The figure shows three views and two pictorial views of one solid part (mm, origin at its lowest corner). Answer the questions. A direction names the side the tool comes from. Coordinates: 2 decimals unless noted, no trailing zeros. Write each loop counter-clockwise with the first axis right and the second up, starting at its lowest first coordinate (ties: lowest second). Pieces come first, ordered by that corner, then holes.
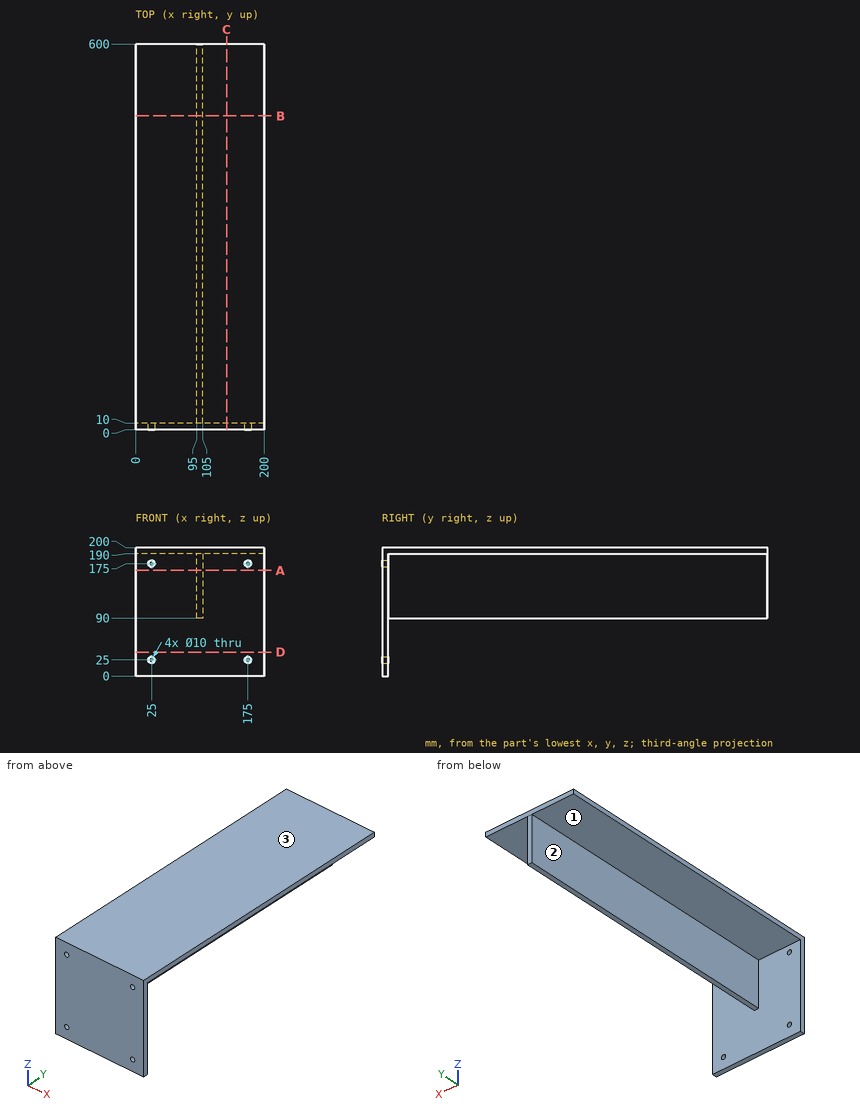
Q1. The part is cut by section B-B, the plane y = 488. Write down the section's boundary in (x, z).
Answers below:
outline: (0, 190) - (95, 190) - (95, 90) - (105, 90) - (105, 190) - (200, 190) - (200, 200) - (0, 200) - close
Q2. Find the intervals of material crossed by probe 1 along Z at (x, y) = (25, 9.8); probe 2 along Y at (x, z) = (163, 98), in increasing order.
Answers below:
probe 1: z = 0 to 20, 30 to 170, 180 to 200
probe 2: y = 0 to 10
Q3. The part is cut by section C-C, the plane x = 142. Write down the section's boundary in (y, z), then the cut area to 3 significant figures.
Answers below:
outline: (0, 0) - (10, 0) - (10, 190) - (600, 190) - (600, 200) - (0, 200) - close
area: 7,900 mm2
Q4. Which of the six approach directions +Z, -Z, +X, -X, +Y, -Y give full straight-line access (tool end or side, diameter ignored) to the marked faces 1, 2 and 3?
Answers below:
face 1: -Z, -X, +Y
face 2: -Z, -X, +Y
face 3: +Z, +X, -X, +Y, -Y
Q5. Given pin 1 (9 mm diameter, centred on x = 175, z = 25, fed in from -Y); pin 2 (5 mm diameter, centred on y = 317, z = 105.5, fed in from -X); pin 3 (8 mm diameter, centred on x = 102, y = 168, fed in from -Z); pin 4 (16 mm diameter, centred on x = 25, z = 25, fed in from +Y), each flat-ended and moving along its own axis, determine where each tip first touches the part or whether it passes through.
Answers below:
pin 1: passes through
pin 2: stops at x = 95
pin 3: stops at z = 90
pin 4: stops at y = 10
Q6. The part is cut by section A-A, the plane z = 164.5. Write down the section's boundary in (x, y).
Answers below:
outline: (0, 0) - (200, 0) - (200, 10) - (105, 10) - (105, 600) - (95, 600) - (95, 10) - (0, 10) - close
Q7. The part is cut by section D-D, the plane z = 37. Write down the section's boundary in (x, y), then the cut area to 3 significant figures.
Answers below:
outline: (0, 0) - (200, 0) - (200, 10) - (0, 10) - close
area: 2,000 mm2
